Verification items for the finished model (mm, model axes). A direction names the side the tool comes from. Give positions to 0.01 mm unless a question says otherwise; leave off trailing zeros. Write each loop counter-clockwise with the first axis right and the second up, starting at its lowest first coordinate (ties: lowest second). Pieces come first, ordered by that corner, then holes.
from build123d import *

# Parameters (mm, degrees)
SKETCH1_R           = 22.5
BOSS_EXTRUDE1_DEPTH = 3.6
SKETCH1_3_R         = 22.5
BOSS_EXTRUDE2_DEPTH = 1
BOSS_EXTRUDE3_DEPTH = 1.6


with BuildPart() as part:
    # Sketch1 → Boss-Extrude1 (new body)
    with BuildSketch(Plane(origin=(0, 0, 0), x_dir=(1, 0, 0), z_dir=(0, 1, 0))):
        Circle(SKETCH1_R)
        with BuildLine():
            Line((-13.65, 11.790472541), (-13.65, 16.290472541))
            Line((-13.65, 16.290472541), (-6.65, 16.290472541))
            Line((-6.65, 16.290472541), (6.65, 16.290472541))
            Line((6.65, 16.290472541), (13.65, 16.290472541))
            Line((13.65, 16.290472541), (13.65, 11.790472541))
            Line((13.65, 11.790472541), (13.65, 4.642529479))
            Line((13.65, 4.642529479), (13.65, -5.41416329))
            ThreePointArc((13.65, -5.41416329), (13.652871179, -5.418313502), (13.65574003, -5.422465323))
            ThreePointArc((13.65574003, -5.422465323), (14.219560095, -14.718302537), (6.25, -19.53666268))
            ThreePointArc((6.25, -19.53666268), (0.055477541, -17.065666548), (-2.737569132, -11.009527459))
            Line((-2.737569132, -11.009527459), (-6.65, -11.009527459))
            Line((-6.65, -11.009527459), (-13.65, -11.009527459))
            Line((-13.65, -11.009527459), (-13.65, -6.509527459))
            Line((-13.65, -6.509527459), (-13.65, 11.790472541))
        make_face(mode=Mode.SUBTRACT)
    extrude(amount=BOSS_EXTRUDE1_DEPTH)

    # Sketch1_3 → Boss-Extrude2 (add)
    with BuildSketch(Plane(origin=(0, 0, 0), x_dir=(1, 0, 0), z_dir=(0, 1, 0))):
        Circle(SKETCH1_3_R)
        with BuildLine():
            Line((-6.65, 11.790472541), (-6.65, 16.290472541))
            Line((-6.65, 16.290472541), (6.65, 16.290472541))
            Line((6.65, 16.290472541), (6.65, 11.790472541))
            Line((6.65, 11.790472541), (13.65, 11.790472541))
            Line((13.65, 11.790472541), (13.65, 4.642529479))
            Line((13.65, 4.642529479), (9.867222257, 4.642529479))
            Line((9.867222257, 4.642529479), (9.867222257, -5.422465323))
            Line((9.867222257, -5.422465323), (13.65, -5.422465323))
            Line((13.65, -5.422465323), (13.65, -5.41416329))
            ThreePointArc((13.65, -5.41416329), (9.158112615, -19.053873551), (-2.737569132, -11.009527459))
            Line((-2.737569132, -11.009527459), (-6.65, -11.009527459))
            Line((-6.65, -11.009527459), (-6.65, -6.509527459))
            Line((-6.65, -6.509527459), (-13.65, -6.509527459))
            Line((-13.65, -6.509527459), (-13.65, 11.790472541))
            Line((-13.65, 11.790472541), (-6.65, 11.790472541))
        make_face(mode=Mode.SUBTRACT)
    extrude(amount=-BOSS_EXTRUDE2_DEPTH)

    # Sketch2 → Boss-Extrude3 (add)
    with BuildSketch(Plane(origin=(0, 0, 0), x_dir=(1, 0, 0), z_dir=(0, 1, 0))):
        with BuildLine():
            Line((-11.7, 13.090472541), (-9.4, 13.090472541))
            ThreePointArc((-9.4, 13.090472541), (-8.622182541, 13.412655081), (-8.3, 14.190472541))
            Line((-8.3, 14.190472541), (-8.3, 14.390472541))
            ThreePointArc((-8.3, 14.390472541), (-8.622182541, 15.16829), (-9.4, 15.490472541))
            Line((-9.4, 15.490472541), (-11.7, 15.490472541))
            ThreePointArc((-11.7, 15.490472541), (-12.477817459, 15.16829), (-12.8, 14.390472541))
            Line((-12.8, 14.390472541), (-12.8, 14.190472541))
            ThreePointArc((-12.8, 14.190472541), (-12.477817459, 13.412655081), (-11.7, 13.090472541))
        make_face()
        with BuildLine():
            Line((-11.7, -10.209527459), (-9.4, -10.209527459))
            ThreePointArc((-9.4, -10.209527459), (-8.622182541, -9.887344919), (-8.3, -9.109527459))
            Line((-8.3, -9.109527459), (-8.3, -8.909527459))
            ThreePointArc((-8.3, -8.909527459), (-8.622182541, -8.13171), (-9.4, -7.809527459))
            Line((-9.4, -7.809527459), (-11.7, -7.809527459))
            ThreePointArc((-11.7, -7.809527459), (-12.477817459, -8.13171), (-12.8, -8.909527459))
            Line((-12.8, -8.909527459), (-12.8, -9.109527459))
            ThreePointArc((-12.8, -9.109527459), (-12.477817459, -9.887344919), (-11.7, -10.209527459))
        make_face()
        with BuildLine():
            Line((11.7, 15.490472541), (9.4, 15.490472541))
            ThreePointArc((9.4, 15.490472541), (8.622182541, 15.16829), (8.3, 14.390472541))
            Line((8.3, 14.390472541), (8.3, 14.190472541))
            ThreePointArc((8.3, 14.190472541), (8.622182541, 13.412655081), (9.4, 13.090472541))
            Line((9.4, 13.090472541), (11.7, 13.090472541))
            ThreePointArc((11.7, 13.090472541), (12.477817459, 13.412655081), (12.8, 14.190472541))
            Line((12.8, 14.190472541), (12.8, 14.390472541))
            ThreePointArc((12.8, 14.390472541), (12.477817459, 15.16829), (11.7, 15.490472541))
        make_face()
    extrude(amount=BOSS_EXTRUDE3_DEPTH)


solid = part.part
Item 1: Set-up check for faces 3 (the face through (-12.469, 0.789, -15.177)), 4 (the face through (11.8, -0.5, -4.643)): record each of +Z, -Z, +X, -X, +Y, -Y from which the full face is reachable in a straight line by a thin tool's end or side.
Answer key:
face 3: +Y
face 4: +Y, -Y
Item 2: Scan lines: line 1 along Z through (x, y) = (18.5, 2.3); line 2 along X through (y, z) = (2.15, 15); line 3 along Y through (x, z) = (-9.5, 10). Record each from-to range of solid material in increasing order.
Answer key:
line 1: z = -12.81 to 12.81
line 2: x = -16.77 to -1.57, 14.07 to 16.77
line 3: y = -1 to 1.6
Item 3: Sectioned sample at D-D on x = 3.5. Record the cut outline in (y, z), then the cut area to 3 significant figures.
Answer key:
outline: (-1, -22.23) - (3.6, -22.23) - (3.6, -16.29) - (-1, -16.29) - close; (-1, 19.11) - (3.6, 19.11) - (3.6, 22.23) - (-1, 22.23) - close
area: 41.7 mm2
Item 4: Sectioned sample at A-A on z = 0. Record the cut outline in (x, y), then the cut area to 3 significant figures.
Answer key:
outline: (-22.5, -1) - (-13.65, -1) - (-13.65, 3.6) - (-22.5, 3.6) - close; (9.87, -1) - (22.5, -1) - (22.5, 3.6) - (13.65, 3.6) - (13.65, 0) - (9.87, 0) - close
area: 85.2 mm2
Item 5: Sectioned sample at C-C on x = -10.5. Record the cut outline in (y, z).
Answer key:
outline: (-1, -19.9) - (3.6, -19.9) - (3.6, -16.29) - (0, -16.29) - (0, -15.49) - (1.6, -15.49) - (1.6, -13.09) - (0, -13.09) - (0, -11.79) - (-1, -11.79) - close; (-1, 6.51) - (0, 6.51) - (0, 7.81) - (1.6, 7.81) - (1.6, 10.21) - (0, 10.21) - (0, 11.01) - (3.6, 11.01) - (3.6, 19.9) - (-1, 19.9) - close
Item 6: Release check for a two-part mould opening along X. For faces 1 (the face through (9, 0, -13)), 2 (the face through (10.382, 1.332, 19.961)) record: released by +X, released by -X, zero draft, split by the parting line, or undercut.
Answer key:
face 1: undercut
face 2: split by the parting line
Item 7: Sectioned sample at B-B on y = 0.8. State how many separate pieces and enclosed holes the cut face has, then the cut area to 3 significant figures.
Answer key:
separate pieces: 4
enclosed holes: 1
area: 749 mm2
Item 8: Depth check by flat-ended pin: pin 1 (3.5 mm diameter, centred on x = -10, z = 9.5, fed in from +Y); pin 2 (1.4 mm diameter, centred on x = -12, z = -14.5, fed in from +Y); pin 3 (0.8 mm diameter, centred on x = -11.5, y = -0.5, fed in from -Z); pin 4 (1 mm diameter, centred on y = 3, z = -3, fed in from -X). Enter the tip coordinate at first touch or a pass-through.
Answer key:
pin 1: stops at y = 3.6
pin 2: stops at y = 1.6
pin 3: stops at z = -19.57
pin 4: stops at x = -22.36
